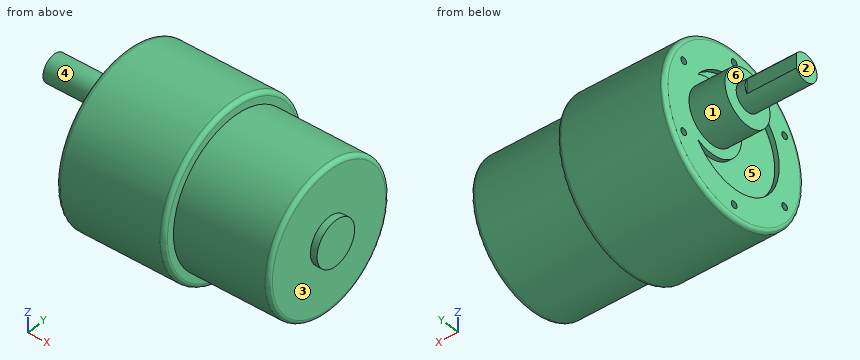
from build123d import *

# Parameters (mm, degrees)
SKETCH2_R           = 6
BOSS_EXTRUDE1_DEPTH = 8
SKETCH3_R           = 2.990422361
BOSS_EXTRUDE2_DEPTH = 13
CUT_EXTRUDE1_DEPTH  = 11
CUT_EXTRUDE2_DEPTH  = 1
SKETCH7_R           = 0.75
CUT_EXTRUDE4_DEPTH  = 2
CIRPATTERN1_COUNT   = 6


with BuildPart() as part:
    # Sketch1 → Revolve2 (revolve)
    with BuildSketch(Plane(origin=(0, 0, 0), x_dir=(1, 0, 0), z_dir=(0, 1, 0))):
        with BuildLine():
            Line((-23.3, 0), (23.5, 0))
            Line((23.5, 0), (23.5, 5))
            Line((23.5, 5), (22, 5))
            Line((22, 5), (22, 15.1))
            ThreePointArc((22, 15.1), (21.736396103, 15.736396103), (21.1, 16))
            Line((21.1, 16), (0.7, 16))
            Line((0.7, 16), (0.7, 17.6))
            ThreePointArc((0.7, 17.6), (0.436396103, 18.236396103), (-0.2, 18.5))
            Line((-0.2, 18.5), (-22.4, 18.5))
            ThreePointArc((-22.4, 18.5), (-23.036396103, 18.236396103), (-23.3, 17.6))
            Line((-23.3, 17.6), (-23.3, 0))
        make_face()
    revolve(axis=Axis((-35.546651827, 0, 0), (1, 0, 0)))

    # Sketch2 → Boss-Extrude1 (add)
    with BuildSketch(Plane.ZY.offset(23.3)):
        with Locations((0, 6)):
            Circle(SKETCH2_R)
    extrude(amount=BOSS_EXTRUDE1_DEPTH)

    # Sketch3 → Boss-Extrude2 (add)
    with BuildSketch(Plane.ZY.offset(31.3)):
        with Locations((0, 6)):
            Circle(SKETCH3_R)
    extrude(amount=BOSS_EXTRUDE2_DEPTH)

    # Sketch5 → Cut-Extrude1 (cut)
    with BuildSketch(Plane.ZY.offset(44.3)):
        with BuildLine():
            Line((-1.6, 8.526385936), (1.6, 8.526385936))
            ThreePointArc((1.6, 8.526385936), (0, 8.990422361), (-1.6, 8.526385936))
        make_face()
    extrude(amount=-CUT_EXTRUDE1_DEPTH, mode=Mode.SUBTRACT)

    # Sketch6 → Cut-Extrude2 (cut)
    with BuildSketch(Plane.ZY.offset(23.3)):
        with BuildLine():
            ThreePointArc((-7.110243003, 9.666666667), (0, -2), (7.110243003, 9.666666667))
            ThreePointArc((7.110243003, 9.666666667), (0, -12), (-7.110243003, 9.666666667))
        make_face()
    extrude(amount=-CUT_EXTRUDE2_DEPTH, mode=Mode.SUBTRACT)

    # Sketch7 → Cut-Extrude4 (cut)
    with BuildSketch(Plane.ZY.offset(23.3)):
        with Locations((15.5, 0)):
            Circle(SKETCH7_R)
    cut_extrude4 = extrude(amount=-CUT_EXTRUDE4_DEPTH, mode=Mode.SUBTRACT)

    # CirPattern1: Cut-Extrude4 ×6 about axis
    cirpattern1_axis = Axis((0, 0, 0), (1, 0, 0))
    for i in range(1, CIRPATTERN1_COUNT):
        add(cut_extrude4.rotate(cirpattern1_axis, i * 360 / CIRPATTERN1_COUNT), mode=Mode.SUBTRACT)


solid = part.part
Can you work these out from the model? Positions are in its coordinate system, mm. Face numbers are marked on the shaded views. A direction names the side the tool comes from. Coordinates: 2 decimals unless noted, no trailing zeros. Order: outer loops, then holes, each group sorted by start corner. A loop starts at its lowest first (then second) coordinate and runs counter-clockwise, first axis right, second up. Notation, with made-up numbers: M 10,-29 L 32,-29 A6 cw 32,-24 Z; hole C -4.5,54.5 d6. An arc over 180 degrees is marked long. Write item = value, one per line.
(1) Suppose I cut it at B-B on x = -12. Please give me the cut outline in (y, z), plus the area to 3 significant figures.
Results are:
outline = C 0,0 d37
area = 1,080 mm2
(2) For pin 1 Ø0.8 at (y, z) = (-13, -7.5) entering from -X; pin 2 Ø8 at (x, z) = (-24.5, -9) entering from -Y; pin 3 Ø0.8 at (y, z) = (13.5, -7.5) entering from -X, each with a flat end and sliding along its axis, tell me the tip position at first contact or that it passes through.
Results are:
pin_1 = -23.3
pin_2 = -17.65
pin_3 = -21.3
(3) If we mould it in two halves opening along Y, with no side actions, what happens to the marked faces 4, 5 and 6? For each: pulls with the +Y half, pulls with the -Y half, needs draft (parallel to the pull), parting line crosses it, or undercut.
Results are:
face_4 = parting line crosses it
face_5 = undercut
face_6 = needs draft
(4) I need wall thicknesses on line 1 along Y through (x, z) = (-21.8, 7.75); line 2 along X through (y, z) = (-0.5, -6); line 3 along Y through (x, z) = (-22.35, 15.5). Which ranges of each line are inside material? Lowest first, please. Write a range as [from, to].
Results are:
line_1 = [-16.8, -14.17], [-12.67, 12.67], [14.17, 16.8]
line_2 = [-22.3, 22]
line_3 = [-10.1, -0.75], [0.75, 10.1]
(5) For the marked faces 1, 2 and 3, which set-ups out of +Z, -Z, +X, -X, +Y, -Y let a thin tool reach every point of the face, with its end or its side?
Results are:
face_1 = -X
face_2 = +Z, -Z, -X, +Y, -Y
face_3 = +X
(6) Suppose I cut it at C-C on x = -38. Please give me the cut outline in (y, z).
Results are:
outline = M 8.53,-1.6 L 8.53,1.6 A2.99 ccw long Z
